```python
from build123d import *

# Parameters (mm, degrees)
CUT_EXTRUDE1_REACH                                   = 90.9
CHAMFER2_SIZE                                        = 1.27
CHAMFER3_SIZE                                        = 1.27
F_38_0_1015_DIAMETER_HOLE1_D                         = 2.5781
F_38_0_1015_DIAMETER_HOLE1_DEPTH                     = 0.254
F_38_0_1015_DIAMETER_HOLE1_TIP                       = 0.774539381
CBORE_FOR_3_8_BINDING_HEAD_MACHINE_SCREW_D           = 10.3124
CBORE_FOR_3_8_BINDING_HEAD_MACHINE_SCREW_DEPTH       = 6.35
CBORE_FOR_3_8_BINDING_HEAD_MACHINE_SCREW_CBORE_D     = 19.05
CBORE_FOR_3_8_BINDING_HEAD_MACHINE_SCREW_CBORE_DEPTH = 1.016
CUT_EXTRUDE3_REACH                                   = 46.45
SKETCH16_R                                           = 5.207
SKETCH16_R_2                                         = 3.3


with BuildPart() as part:
    # Sketch1 → Revolve1 (revolve)
    with BuildSketch(Plane(origin=(0, 0, 0), x_dir=(0, 0, -1), z_dir=(1, 0, 0))):
        Polygon((10.16, 0), (16.51, 0), (16.51, -44.45), (-27.94, -44.45), (-27.94, -38.1), (-25.4, -38.1), (-25.4, -39.878), (-21.844, -39.878), (-21.844, -38.1), (-0.508, -38.1), (-0.508, -36.83), (10.16, -36.83), align=None)
    revolve(axis=Axis((0, 0, 77.403157895), (0, 0, -1)))

    # Sketch2 → Cut-Extrude1 (cut, up to next)
    with BuildSketch(Plane(origin=(0, 44.45, 0), x_dir=(1, 0, 0), z_dir=(0, 1, 0)), mode=Mode.PRIVATE) as cut_extrude1_sk1:
        with BuildLine():
            Line((-6.35, -27.94), (6.35, -27.94))
            Line((6.35, -27.94), (6.35, -25.1968))
            ThreePointArc((6.35, -25.1968), (5.42006403, -22.95173597), (3.175, -22.0218))
            Line((3.175, -22.0218), (-3.175, -22.0218))
            ThreePointArc((-3.175, -22.0218), (-5.42006403, -22.95173597), (-6.35, -25.1968))
            Line((-6.35, -25.1968), (-6.35, -27.94))
        make_face()
    cut_extrude1_tool1 = extrude(cut_extrude1_sk1.sketch, amount=-CUT_EXTRUDE1_REACH, mode=Mode.PRIVATE) & part.part
    add(cut_extrude1_tool1.solids().sort_by_distance((0, 44.45, 25.118327))[0], mode=Mode.SUBTRACT)

    # Chamfer2
    chamfer2_edges = [part.edges().sort_by_distance(p)[0] for p in [
        (0, 44.45, -16.51),
        (-44.335876123, -3.183172689, 27.94),
    ]]
    chamfer(chamfer2_edges, length=CHAMFER2_SIZE)

    # Chamfer3
    chamfer3_edges = [part.edges().sort_by_distance(p)[0] for p in [
        (0, -38.1, 27.94),
    ]]
    chamfer(chamfer3_edges, length=CHAMFER3_SIZE)

    # #38 (0.1015) Diameter Hole1
    with Locations(Plane.XY.offset(-10.16)):
        with Locations((0, 0)):
            Hole(F_38_0_1015_DIAMETER_HOLE1_D / 2, depth=F_38_0_1015_DIAMETER_HOLE1_DEPTH)
            with Locations((0, 0, -(F_38_0_1015_DIAMETER_HOLE1_DEPTH + F_38_0_1015_DIAMETER_HOLE1_TIP / 2))):  # 118° drill point
                Cone(0, F_38_0_1015_DIAMETER_HOLE1_D / 2, F_38_0_1015_DIAMETER_HOLE1_TIP, mode=Mode.SUBTRACT)

    # CBORE for 3/8 Binding Head Machine Screw1
    with Locations(Plane(origin=(0, 0, -16.51), x_dir=(-1, 0, 0), z_dir=(0, 0, -1))):
        with Locations((-24.13512246, 0)):
            CounterBoreHole(CBORE_FOR_3_8_BINDING_HEAD_MACHINE_SCREW_D / 2, CBORE_FOR_3_8_BINDING_HEAD_MACHINE_SCREW_CBORE_D / 2, CBORE_FOR_3_8_BINDING_HEAD_MACHINE_SCREW_CBORE_DEPTH, depth=CBORE_FOR_3_8_BINDING_HEAD_MACHINE_SCREW_DEPTH)

    # Sketch16 → Cut-Extrude3 (cut, up to next)
    with BuildSketch(Plane(origin=(0, 0, -16.51), x_dir=(-1, 0, 0), z_dir=(0, 0, -1)), mode=Mode.PRIVATE) as cut_extrude3_sk1:
        with Locations((0.800871739, -13.932849809)):
            Circle(SKETCH16_R)
    cut_extrude3_tool1 = extrude(cut_extrude3_sk1.sketch, amount=-CUT_EXTRUDE3_REACH, mode=Mode.PRIVATE) & part.part
    add(cut_extrude3_tool1.solids().sort_by_distance((-0.800872, -13.93285, -16.51))[0], mode=Mode.SUBTRACT)
    # Sketch16 → Cut-Extrude3 (cut, up to next)
    with BuildSketch(Plane(origin=(0, 0, -16.51), x_dir=(-1, 0, 0), z_dir=(0, 0, -1)), mode=Mode.PRIVATE) as cut_extrude3_sk2:
        with Locations((6.332326955, 14.108828715)):
            Circle(SKETCH16_R_2)
    cut_extrude3_tool2 = extrude(cut_extrude3_sk2.sketch, amount=-CUT_EXTRUDE3_REACH, mode=Mode.PRIVATE) & part.part
    add(cut_extrude3_tool2.solids().sort_by_distance((-6.332327, 14.108829, -16.51))[0], mode=Mode.SUBTRACT)


solid = part.part
```
Read the model definition and answer for the solid it produces. Units are mm, in the model's axes. A direction names the side the tool comes from. Round coordinates to 2 decimals unless told otherwise and drop trailing zeros. Loops run counter-clockwise (first coordinate to the right, second up) from the corner with the lowest first, then second, coordinate; pieces in that order, holes last. Notation, with made-up numbers: (39, 41) -> (86, 41) arc R20 cw to (86, 74) -> close; hole circle Ø10 at (33, -19.75). An arc over 180 degrees is marked (long way). One line per item, written item: value.
1) Consider L1, parallel to X at y = 0, z = 4; L2, parallel to Y at x = 0, z = -2. Determine where each line is inside the solid, lowest interval first. Write a range as [from, to].
Answer list:
L1: x = [-44.45, -38.1], [38.1, 44.45]
L2: y = [-44.45, -36.83], [36.83, 44.45]
2) A cutting plane is placed at A-A (z = -5). Determine the outline of the cut face in (x, y), and give its area (3 significant figures).
Answer list:
outline: circle Ø88.9 at (0, 0); hole circle Ø73.66 at (0, 0)
area: 1,950 mm²
3) For faces 5 (the face through (6.35, 41, 27)), 6 (the face through (23.183, 30.235, 11.027)), 7 (the face through (-0.12, -8.77, -13.38)), 8 (the face through (-11.978, -38.037, 23.597)), 9 (the face through (20, -4, -15.494)), determine the directions among +Z, -Z, +X, -X, +Y, -Y from which every point of the face is accessible in a straight line to the end or side of a thin tool.
Answer list:
face 5: +Z, +Y
face 6: +Z
face 7: +Z, -Z
face 8: none
face 9: -Z
4) The mould has two halves that part along Z. Classify faces 1 (the face through (22.41, 29.227, -4.901)), 2 (the face through (20.5, -32.3, 21.844)), 3 (the face through (-31.2, 19.9, 0.508)), 4 (the face through (-1, -1, -16.51)): pulls with the +Z half, pulls with the -Z half, needs draft (parallel to the pull), parting line crosses it, or undercut.
Answer list:
face 1: needs draft
face 2: undercut
face 3: pulls with the +Z half
face 4: pulls with the -Z half
5) A cutting plane is placed at B-B (z = 7). Determine the outline of the cut face in (x, y), and give its area (3 significant figures).
Answer list:
outline: circle Ø88.9 at (0, 0); hole circle Ø76.2 at (0, 0)
area: 1,650 mm²
6) Flat-ended cylindrical pins translate along their axes: P1, Ø22, axis at x = -2, y = -17.5, coming from the +Z side; P2, Ø10, axis at y = 22.5, z = 13, coming from the +X side; P3, Ø6, axis at y = 7, z = 8.5, coming from the +X side. Find the tip coordinate at first contact, or state that the pin passes through.
Answer list:
P1: stops at z = -10.16
P2: stops at x = 40.86
P3: stops at x = 44.27
